```python
from build123d import *

# Parameters (mm, degrees)
BOSS_EXTRUDE1_DEPTH = 10
SKETCH2_R           = 3
BOSS_EXTRUDE2_DEPTH = 2.5
CUT_EXTRUDE1_DEPTH  = 10


with BuildPart() as part:
    # Sketch1 → Boss-Extrude1 (new body)
    with BuildSketch(Plane(origin=(0, 0, 0), x_dir=(1, 0, 0), z_dir=(0, 1, 0))):
        with BuildLine():
            Line((-22.931089862, 8.626419753), (-14.975405624, 5.633580247))
            ThreePointArc((-14.975405624, 5.633580247), (0, 16), (14.975405624, 5.633580247))
            Line((14.975405624, 5.633580247), (22.931089862, 8.626419753))
            ThreePointArc((22.931089862, 8.626419753), (0, 24.5), (-22.931089862, 8.626419753))
        make_face()
    extrude(amount=BOSS_EXTRUDE1_DEPTH)

    # Sketch2 → Boss-Extrude2 (add)
    with BuildSketch(Plane.XZ):
        with BuildLine():
            Line((76.870427411, -16), (76.870427411, 16))
            Line((76.870427411, 16), (21.748563171, 16))
            ThreePointArc((21.748563171, 16), (12.186057607, 24.093567606), (0, 27))
            ThreePointArc((0, 27), (-27, 0), (0, -27))
            ThreePointArc((0, -27), (12.186057607, -24.093567606), (21.748563171, -16))
            Line((21.748563171, -16), (76.870427411, -16))
        make_face()
        with Locations(Location((0, 0, 0), (0, 0, 270))):
            Circle(SKETCH2_R, mode=Mode.SUBTRACT)
    extrude(amount=BOSS_EXTRUDE2_DEPTH)

    # Sketch3 → Cut-Extrude1 (cut)
    with BuildSketch(Plane(origin=(0, 0, 0), x_dir=(1, 0, 0), z_dir=(0, 1, 0))):
        with BuildLine():
            Line((76.870427411, 16), (60.870427411, 16))
            ThreePointArc((60.870427411, 16), (72.184135957, 11.313708452), (76.870427411, -1.33e-07))
            Line((76.870427411, -1.33e-07), (76.870427411, 16))
        make_face()
        with BuildLine():
            Line((76.870427411, -16), (76.870427411, -1.33e-07))
            ThreePointArc((76.870427411, -1.33e-07), (72.184135863, -11.313708546), (60.870427411, -16))
            Line((60.870427411, -16), (76.870427411, -16))
        make_face()
    extrude(amount=-CUT_EXTRUDE1_DEPTH, mode=Mode.SUBTRACT)


solid = part.part
```
The listing builds one solid part. Answer for the finished solid, in the listing's coordinates (mm). A direction names the side the tool comes from. Round coordinates to 2 decimals unless told otherwise and drop trailing zeros. Write each loop counter-clockwise with the first axis right and the second up, starting at its lowest first coordinate (ties: lowest second). Pieces come first, ordered by that corner, then holes. Notation, with made-up numbers: (8.25, -17) -> (34.25, -17) arc R20 ccw to (34.25, 12) -> close; hole circle Ø4 at (46, 80). An arc over 180 degrees is marked (long way). Answer as a JSON object with one key per item and string values. Group by question number.
Q1. Which of the six approach directions +Z, -Z, +X, -X, +Y, -Y give full straight-line access (tool end or side, diameter ignored) to faces 1 (the face through (-19.01, 4.93, -7.15)), 2 (the face through (41, -1, -16)), 3 (the face through (42, -1, 16)), 4 (the face through (18.9, 4.93, -7.11))?
Q2. Each of these flat-tipped pins is pushed along its axis until it touches: pin 1 Ø0.8 at (x, y) = (48.5, -1) entering from +Z; pin 2 Ø16 at (x, z) = (15.5, 5.5) entering from +Y; pin 3 Ø0.8 at (x, y) = (37.5, -1) entering from -Z. Where does it stop, or does it pass through?
Q3. Section B-B (z = -11) is taken. Write down the section's boundary in (x, y).
Q4. Section A-A (x = 26) is taken. Write down the section's boundary in (y, z), plus the area to 3 significant figures.
Q5. Straight lines are drawn through the part: line 1 along Y through (x, z) = (-0.5, 7.5); line 2 along X through (y, z) = (6, -9); line 3 along Z through (x, y) = (-17, 5.5). For each, find the intervals that lie inside material, in ascending order.
Q6. Section C-C (y = 5.5) is taken. Write down the section's boundary in (x, z).
Check values:
{
 "1": {"face 1": "+Z, -X, +Y", "face 2": "-Z, +X, +Y, -Y", "face 3": "+Z, +X, +Y, -Y", "face 4": "+Z, +X, +Y"},
 "2": {"pin 1": "z = 16", "pin 2": "y = 0", "pin 3": "z = -16"},
 "3": {"outline": "(-24.66, -2.5) -> (72.49, -2.5) -> (72.49, 0) -> (21.89, 0) -> (21.89, 10) -> (11.62, 10) -> (11.62, 0) -> (-11.62, 0) -> (-11.62, 10) -> (-21.89, 10) -> (-21.89, 0) -> (-24.66, 0) -> close"},
 "4": {"outline": "(-2.5, -16) -> (0, -16) -> (0, 16) -> (-2.5, 16) -> close", "area": "80.0 mm^2"},
 "5": {"line 1": "-2.5 to 0", "line 2": "-22.79 to -13.23, 13.23 to 22.79", "line 3": "-17.64 to -6.4"},
 "6": {"outline": "(-22.93, -8.63) arc R24.5 ccw to (22.93, -8.63) -> (14.98, -5.63) arc R16 cw to (-14.98, -5.63) -> close"}
}
